For this review, take the finished solid that the model builds, in its own axes (mm). A direction names the side the tool comes from. Give positions to 0.01 mm unless a question says otherwise; leave off trailing zeros. Loops run counter-clockwise (first coordinate to the right, second up) from the corner with the lowest first, then second, coordinate; pieces in that order, holes last. Notation, with made-up numbers: (-39.75, 44) - (4.25, 44) arc R13 cw to (4.25, 59) - close; hole circle Ø8 at (-7.75, 78.5). An arc over 180 degrees is marked (long way). Use CSV: the item, a comma, the result in double quotes. Start each with the question number.
1. Wall thickness on line 1 (Y direction, x = 420.5, z = 15); line 2 (Z direction, x = 548.5, y = -10.5): over which ranges is each line inside the solid? List them lowest first.
2. Take a section at C-C on x = 98. Give the boundary of the cut face in (y, z), plus the area to 3 significant figures.
3. Take a section at B-B on z = -8.5. Give the boundary of the cut face in (x, y).
4. Take a section at A-A on y = 4.5. Give the boundary of the cut face in (x, z), plus the area to 3 significant figures.
5. Mouldability with a two-part tool opening along Y and no side actions: class faces 1 (the flat face through (616, -32.5, 0)), 2 (the flat face through (616, -37.5, 0)), 3 (the flat face through (616, 37.5, 0)), 4 (the flat face through (616, -1, -35)) as pulls with the +Y half, pulls with the -Y half, needs draft (parallel to the pull), parting line crosses it, or undercut.
6. For faces 5 (the flat face through (616, -1, 35)), 6 (the flat face through (616, 0, 30)), list the 3-axis set-ups (+Z, -Z, +X, -X, +Y, -Y) from which the entire face can be reached by the end or side of a thin tool; tool diameter is ignored.
```python
from build123d import *

# Parameters (mm, degrees)
SKETCH_2_W      = 70
SKETCH_2_H      = 75
SKETCH_2_W_2    = 60
SKETCH_2_H_2    = 65
EXTRUDE_1_DEPTH = 1250


with BuildPart() as part:
    # Эскиз2 → Вытянуть-Тонкостенный1 (new body)
    with BuildSketch(Plane(origin=(0, 0, 0), x_dir=(0, 0, -1), z_dir=(1, 0, 0))):
        Rectangle(SKETCH_2_W, SKETCH_2_H)
        Rectangle(SKETCH_2_W_2, SKETCH_2_H_2, mode=Mode.SUBTRACT)
    extrude(amount=EXTRUDE_1_DEPTH)


solid = part.part
```
Check result:
1,line 1,"y = -37.5 to -32.5, 32.5 to 37.5"
1,line 2,"z = -35 to -30, 30 to 35"
2,outline,"(-37.5, -35) - (37.5, -35) - (37.5, 35) - (-37.5, 35) - close; hole (-32.5, -30) - (32.5, -30) - (32.5, 30) - (-32.5, 30) - close"
2,area,"1,350 mm²"
3,outline,"(0, -37.5) - (1250, -37.5) - (1250, -32.5) - (0, -32.5) - close; (0, 32.5) - (1250, 32.5) - (1250, 37.5) - (0, 37.5) - close"
4,outline,"(0, -35) - (1250, -35) - (1250, -30) - (0, -30) - close; (0, 30) - (1250, 30) - (1250, 35) - (0, 35) - close"
4,area,"12,500 mm²"
5,face 1,"undercut"
5,face 2,"pulls with the -Y half"
5,face 3,"pulls with the +Y half"
5,face 4,"needs draft"
6,face 5,"+Z, +X, -X, +Y, -Y"
6,face 6,"+X, -X"
